from build123d import *

# Parameters (mm, degrees)
F0_R     = 11.2
F1_DEPTH = 25


with BuildPart() as f1:
    # F0 (on Top) → F1 (new body)
    with BuildSketch(Plane.XY):
        with BuildLine():
            ThreePointArc((0.281874, 11.196452), (8.018634, 7.819303), (11.2, 0))
            ThreePointArc((11.2, 0), (10.853993, -2.762398), (9.837349, -5.354116))
            ThreePointArc((9.837349, -5.354116), (13.358937, -1.523251), (18.087433, 0.648944))
            ThreePointArc((18.087433, 0.648944), (11.142377, 7.574406), (11.184069, 17.382265))
            ThreePointArc((11.184069, 17.382265), (6.514064, 12.912721), (0.281874, 11.196452))
        make_face()
        with BuildLine():
            ThreePointArc((-0.281874, 11.196452), (0, 11.2), (0.281874, 11.196452))
            ThreePointArc((0.281874, 11.196452), (6.514064, 12.912721), (11.184069, 17.382265))
            ThreePointArc((11.184069, 17.382265), (12.68601, 20.74582), (13.2, 24.393442))
            ThreePointArc((13.2, 24.393442), (-4.87055, 36.66201), (-9.605719, 15.339705))
            ThreePointArc((-9.605719, 15.339705), (-5.360295, 12.330804), (-0.281874, 11.196452))
        make_face()
        with Locations((0, 24.393442)):
            Circle(F0_R, mode=Mode.SUBTRACT)
        with BuildLine():
            ThreePointArc((18.087433, 0.648944), (13.358937, -1.523251), (9.837349, -5.354116))
            ThreePointArc((9.837349, -5.354116), (9.699485, -5.6), (9.555475, -5.842337))
            ThreePointArc((9.555475, -5.842337), (7.925712, -12.097705), (9.461449, -18.37682))
            ThreePointArc((9.461449, -18.37682), (24.309413, -25.006939), (34.325341, -12.196721))
            ThreePointArc((34.325341, -12.196721), (29.314957, -1.844418), (18.087433, 0.648944))
        make_face()
        with Locations((21.125341, -12.196721)):
            Circle(F0_R, mode=Mode.SUBTRACT)
        with BuildLine():
            ThreePointArc((-9.837349, -5.354116), (-9.699485, 5.6), (-0.281874, 11.196452))
            ThreePointArc((-0.281874, 11.196452), (-5.360295, 12.330804), (-9.605719, 15.339705))
            ThreePointArc((-9.605719, 15.339705), (-12.130817, 5.862379), (-20.645517, 0.994555))
            ThreePointArc((-20.645517, 0.994555), (-14.439776, -0.815015), (-9.837349, -5.354116))
        make_face()
        with BuildLine():
            ThreePointArc((9.461449, -18.37682), (7.925712, -12.097705), (9.555475, -5.842337))
            ThreePointArc((9.555475, -5.842337), (0, -11.2), (-9.555475, -5.842337))
            ThreePointArc((-9.555475, -5.842337), (-8.339368, -8.916647), (-7.925341, -12.196721))
            ThreePointArc((-7.925341, -12.196721), (-8.065175, -14.112985), (-8.481715, -15.988649))
            ThreePointArc((-8.481715, -15.988649), (0.98844, -13.436785), (9.461449, -18.37682))
        make_face()
        with BuildLine():
            ThreePointArc((-9.555475, -5.842337), (-9.699485, -5.6), (-9.837349, -5.354116))
            ThreePointArc((-9.837349, -5.354116), (-14.439776, -0.815015), (-20.645517, 0.994555))
            ThreePointArc((-20.645517, 0.994555), (-31.856768, -19.882843), (-8.481715, -15.988649))
            ThreePointArc((-8.481715, -15.988649), (-8.065175, -14.112985), (-7.925341, -12.196721))
            ThreePointArc((-7.925341, -12.196721), (-8.339368, -8.916647), (-9.555475, -5.842337))
        make_face()
        with Locations((-21.125341, -12.196721)):
            Circle(F0_R, mode=Mode.SUBTRACT)
    extrude(amount=F1_DEPTH)


solid = f1.part
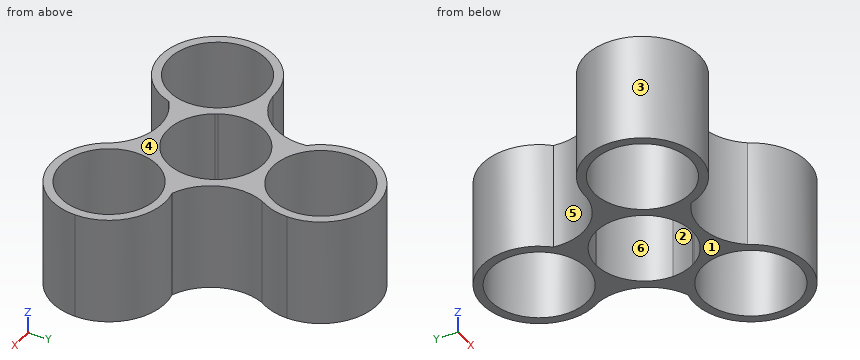
Geometry check sheet. Reference: the model listing, model coordinates, mm. Face numbers are marked on the shaded views. A direction names the side the tool comes from. Coordinates: 2 decimals unless noted, no trailing zeros. Loops run counter-clockwise (first coordinate to the right, second up) from the corner with the lowest first, then second, coordinate; pieces in that order, holes last. Notation, with made-up numbers: (50, -36.5) - (95, -36.5) arc R16 cw to (95, -26.5) - close; hole circle Ø9 at (69, 62). An arc over 180 degrees is marked (long way). Use one line per item in the form item = value. Start each with the question number.
Item 1: Tool access check on the marked faces 1 and 2. Record the directions out of +Z, -Z, +X, -X, +Y, -Y that give a thin tool (end or side, any length) a straight path to the whole face; none if there is none.
Item 2: Section check C-C, the plane y = 9.5. Enter the section's corners in (x, z).
Item 3: Section check D-D, the plane z = 4. Enter the section's corners in (x, y), and give its area (3 significant figures).
Item 4: Thickness scan on probe 1 along Y at (x, z) = (0, 7.75); probe 2 along Y at (x, z) = (21, 18.25); probe 3 along X at (y, z) = (-18.5, 2.5). Record the ranges inside material, lowest first.
Item 5: Section check A-A, the plane x = -17.5. Enter the section's corners in (y, z).
Item 6: Mould release check, pull along X, two halves, no side actions. Record for the marked faces 3, 4, 5 and 6: +X half, -X half, draft (parallel to the pull), parting line (faces both ways), or undercut.
Item 7: Section check B-B, the plane y = -10. Enter the section's corners in (x, z), and give its area (3 significant figures).
Item 8: Gauge pin test, flat ends, axial feed: pin 1 (10 mm diameter, centred on y = 2, z = 19, fed in from +X); pin 2 (1 mm diameter, centred on x = -26, z = 18, fed in from +Y); pin 3 (4 mm diameter, centred on x = -13.5, z = 3.5, fed in from -Y); pin 4 (13.5 mm diameter, centred on x = 0, y = 24.39, fed in from +Z). Record the tip position at first contact, or that the pin passes through.
Computed:
q1.face_1 = -Z, +X, -X, +Y, -Y
q1.face_2 = +Z, -Z
q2.outline = (-10.18, 0) - (-5.93, 0) - (-5.93, 25) - (-10.18, 25) - close; (5.93, 0) - (10.52, 0) - (10.52, 25) - (5.93, 25) - close
q3.outline = (-20.65, 0.99) arc R13.2 ccw (long way) to (-8.48, -15.99) arc R12.73 cw to (9.46, -18.38) arc R13.2 ccw (long way) to (18.09, 0.65) arc R12.73 cw to (11.18, 17.38) arc R13.2 ccw to (13.2, 24.39) arc R13.2 ccw (long way) to (-9.61, 15.34) arc R12.73 cw to start; hole circle Ø22.4 at (-21.13, -12.2); hole circle Ø22.4 at (0, 24.39); hole (-9.84, -5.35) arc R11.2 ccw to (-9.56, -5.84) arc R11.2 ccw to (9.56, -5.84) arc R11.2 ccw to (9.84, -5.35) arc R11.2 ccw to (11.2, 0) arc R11.2 ccw to (0.28, 11.2) arc R11.2 ccw to (-0.28, 11.2) arc R11.2 ccw to start; hole circle Ø22.4 at (21.13, -12.2)
q3.area = 669 mm2
q4.probe_1 = -13.34 to -11.2, 11.2 to 13.19, 35.59 to 37.59
q4.probe_2 = -25.4 to -23.4, -1 to 1
q4.probe_3 = -32.72 to -30.38, -11.87 to -9.53, 9.53 to 11.87, 30.38 to 32.72
q5.outline = (-24.89, 0) - (-22.79, 0) - (-22.79, 25) - (-24.89, 25) - close; (-1.6, 0) - (1.8, 0) - (1.8, 25) - (-1.6, 25) - close
q6.face_3 = undercut
q6.face_4 = draft
q6.face_5 = -X half
q6.face_6 = undercut
q7.outline = (-34.14, 0) - (-32.11, 0) - (-32.11, 25) - (-34.14, 25) - close; (-10.14, 0) - (-5.04, 0) - (-5.04, 25) - (-10.14, 25) - close; (5.04, 0) - (10.14, 0) - (10.14, 25) - (5.04, 25) - close; (32.11, 0) - (34.14, 0) - (34.14, 25) - (32.11, 25) - close
q7.area = 357 mm2
q8.pin_1 = 30.59
q8.pin_2 = 0.26
q8.pin_3 = -24.14
q8.pin_4 = through
